from build123d import *

# Parameters (mm, degrees)
SKETCH5_W           = 26
SKETCH5_H           = 26
BOSS_EXTRUDE1_DEPTH = 10
SKETCH4_R           = 10.75
CUT_EXTRUDE1_DEPTH  = 4
SKETCH6_W           = 10
SKETCH6_H           = 3.483566845
CUT_EXTRUDE2_DEPTH  = 4
LPATTERN1_COUNT     = 8
LPATTERN1_PITCH     = 26
SKETCH7_W           = 10
SKETCH7_H           = 4
CUT_EXTRUDE3_DEPTH  = 183.737516674
SKETCH12_W          = 208
SKETCH12_H          = 10
BOSS_EXTRUDE3_DEPTH = 20
SKETCH14_W          = 46
SKETCH14_H          = 10
BOSS_EXTRUDE4_DEPTH = 20
SKETCH15_W          = 46
SKETCH15_H          = 20
BOSS_EXTRUDE5_DEPTH = 45
SKETCH16_W          = 20
SKETCH16_H          = 5
CUT_EXTRUDE5_DEPTH  = 20
SKETCH17_R          = 6
CUT_EXTRUDE6_DEPTH  = 45
SKETCH18_W          = 6
SKETCH18_H          = 19
CUT_EXTRUDE7_DEPTH  = 20
SNAP_START          = 2.145910006
SNAP_HOOK1_DEPTH    = 13
FILLET2_R           = 2


# Read off the part's stored shape, not the designer's step: Snap Hook1
with BuildPart() as part:
    # Sketch5 → Boss-Extrude1 (new body)
    with BuildSketch(Plane(origin=(0, 0, 0), x_dir=(1, 0, 0), z_dir=(0, 1, 0))):
        Rectangle(SKETCH5_W, SKETCH5_H)
    boss_extrude1 = extrude(amount=-BOSS_EXTRUDE1_DEPTH)

    # Sketch4 → Cut-Extrude1 (cut)
    with BuildSketch(Plane(origin=(0, 0, 0), x_dir=(1, 0, 0), z_dir=(0, 1, 0))):
        with Locations(Location((0, 0, 0), (0, 0, 270))):
            Circle(SKETCH4_R)
    cut_extrude1 = extrude(amount=-CUT_EXTRUDE1_DEPTH, mode=Mode.SUBTRACT)

    # Sketch6 → Cut-Extrude2 (cut)
    with BuildSketch(Plane(origin=(0, 0, 0), x_dir=(1, 0, 0), z_dir=(0, 1, 0))):
        with Locations((0, 11.258216578)):
            Rectangle(SKETCH6_W, SKETCH6_H)
    cut_extrude2 = extrude(amount=-CUT_EXTRUDE2_DEPTH, mode=Mode.SUBTRACT)

    # LPattern1: Boss-Extrude1, Cut-Extrude1, Cut-Extrude2 ×8
    with Locations(*[(0, 0, -i * LPATTERN1_PITCH) for i in range(1, LPATTERN1_COUNT)]):
        add(boss_extrude1)
        add(cut_extrude1, mode=Mode.SUBTRACT)
        add(cut_extrude2, mode=Mode.SUBTRACT)

    # Sketch7 → Cut-Extrude3 (cut, through all)
    with BuildSketch(Plane.XY.offset(-13)):
        with Locations((0, -2)):
            Rectangle(SKETCH7_W, SKETCH7_H)
    extrude(amount=-CUT_EXTRUDE3_DEPTH, mode=Mode.SUBTRACT)

    # Sketch12 → Boss-Extrude3 (add)
    with BuildSketch(Plane(origin=(13, 0, 0), x_dir=(0, 0, -1), z_dir=(1, 0, 0))):
        with Locations((91, -5)):
            Rectangle(SKETCH12_W, SKETCH12_H)
    extrude(amount=BOSS_EXTRUDE3_DEPTH)

    # Sketch14 → Boss-Extrude4 (add)
    with BuildSketch(Plane(origin=(0, 0, -195), x_dir=(-1, 0, 0), z_dir=(0, 0, -1))):
        with Locations((-10, -5)):
            Rectangle(SKETCH14_W, SKETCH14_H)
    extrude(amount=BOSS_EXTRUDE4_DEPTH)

    # Sketch15 → Boss-Extrude5 (add)
    with BuildSketch(Plane(origin=(0, 0, 0), x_dir=(1, 0, 0), z_dir=(0, 1, 0))):
        with Locations((10, 205)):
            Rectangle(SKETCH15_W, SKETCH15_H)
    extrude(amount=BOSS_EXTRUDE5_DEPTH)

    # Sketch16 → Cut-Extrude5 (cut)
    with BuildSketch(Plane(origin=(0, 0, -215), x_dir=(-1, 0, 0), z_dir=(0, 0, -1))):
        with Locations((0, -1.5)):
            Rectangle(SKETCH16_W, SKETCH16_H)
    extrude(amount=-CUT_EXTRUDE5_DEPTH, mode=Mode.SUBTRACT)

    # Sketch17 → Cut-Extrude6 (cut)
    with BuildSketch(Plane(origin=(0, 0, -215), x_dir=(-1, 0, 0), z_dir=(0, 0, -1))):
        with Locations((-0.602201255, 14)):
            Circle(SKETCH17_R)
    extrude(amount=-CUT_EXTRUDE6_DEPTH, mode=Mode.SUBTRACT)

    # Sketch18 → Cut-Extrude7 (cut)
    with BuildSketch(Plane.ZY.offset(13)):
        with Locations((-207, 13.5)):
            Rectangle(SKETCH18_W, SKETCH18_H)
    extrude(amount=-CUT_EXTRUDE7_DEPTH, mode=Mode.SUBTRACT)

    # Snap Hook1 outline → Snap Hook1 (add)
    with BuildSketch(Plane.YZ.offset(SNAP_START)):
        Polygon((45, -207.281762619), (65, -207.281762619), (65, -209.025762619), (71, -207.281762619), (71, -205.531762619), (45, -202.281762619), align=None)
    extrude(amount=SNAP_HOOK1_DEPTH)

    # Fillet2
    fillet2_edges = [part.edges().sort_by_distance(p)[0] for p in [
        (10, -10, -215),
        (10, -10, 13),
    ]]
    fillet(fillet2_edges, radius=FILLET2_R)


solid = part.part
The model under review builds one solid part; all positions refer to its coordinate system, in mm. A direction names the side the tool comes from. Round coordinates to 2 decimals unless told otherwise and drop trailing zeros. Loops run counter-clockwise (first coordinate to the right, second up) from the corner with the lowest first, then second, coordinate; pieces in that order, holes last. Notation, with made-up numbers: M -38,42 L -25,42 A4 cw -25,46 Z; hole C -39,86 d4. An arc over 180 degrees is marked long. Answer as CSV lines item,"result". Start each with the question number.
Item 1: For faces 1 (the face through (-10.75, -1.97, -26.16)), 2 (the face through (7, 14, -207)), 3 (the face through (0, 1, -205)), 4 (the face through (2.146, 55, -206)), list the 3-axis set-ups (+Z, -Z, +X, -X, +Y, -Y) from which the entire face can be reached by the end or side of a thin tool; tool diameter is ignored.
Item 2: Consider section B-B (x = 19.5). Write out the cut boundary in (y, z).
Item 3: Mouldability with a two-part tool opening along Y and no side actions: class faces 5 (the face through (15, 0, -90)), 6 (the face through (10.75, -1.97, -103.84)), 7 (the face through (10, -2, -205)) as released by +Y, released by -Y, zero draft, split by the parting line, or undercut.
Item 4: Wall thickness on line 1 (X direction, y = -0.95, z = 0); line 2 (Y direction, x = -2.5, z = -135.5); line 3 (Z direction, x = -5, y = 20): over which ranges is each line inside the solid? List them lowest first. Write a range as [from, to].
Item 5: Insertion check: P1, Ø3, axis at y = 14, z = -207, coming from the -X side; P2, Ø24.5, axis at x = 0, z = 0, coming from the +Y side; P3, Ø4, axis at x = -2, y = 43, coming from the +Z side. Each pin has a flat end and moves straight along its axis. Give the tip position at first contact, or say it passes through.
Item 6: Consider section D-D (x = 0). Write out the cut boundary in (y, z).
Item 7: Consider section A-A (y = 14). Write out the cut boundary in (x, z).
Item 8: Consider section C-C (z = 0). Write out the cut boundary in (x, y).
Answer:
1,face 1,"+Y"
1,face 2,"-X"
1,face 3,"+Z, -Z"
1,face 4,"+Z, -Z, -X, +Y"
2,outline,"M -10,-213 A2 ccw -8,-215 L 45,-215 L 45,-195 L 0,-195 L 0,13 L -8,13 A2 ccw -10,11 Z"
3,face 5,"released by +Y"
3,face 6,"zero draft"
3,face 7,"undercut"
4,line 1,"x = [-13, -10.75], [10.75, 33]"
4,line 2,"y = [-10, -4]"
4,line 3,"z = [-215, -210], [-204, -195]"
5,P1,"stops at x = 7"
5,P2,"stops at y = 0"
5,P3,"stops at z = -195"
6,outline,"M -10,-213 A2 ccw -8,-215 L -4,-215 L -4,10.75 L 0,10.75 L 0,13 L -8,13 A2 ccw -10,11 Z; M 1,-215 L 8.03,-215 L 8.03,-210 L 4,-210 L 4,-204 L 8.03,-204 L 8.03,-195 L 1,-195 Z; M 19.97,-215 L 45,-215 L 45,-195 L 19.97,-195 L 19.97,-204 L 23,-204 L 23,-210 L 19.97,-210 Z"
7,outline,"M -13,-215 L -5.4,-215 L -5.4,-210 L -13,-210 Z; M -13,-204 L -5.4,-204 L -5.4,-195 L -13,-195 Z; M 6.6,-215 L 33,-215 L 33,-195 L 6.6,-195 L 6.6,-204 L 7,-204 L 7,-210 L 6.6,-210 Z"
8,outline,"M -13,-10 L 33,-10 L 33,0 L 10.75,0 L 10.75,-4 L -10.75,-4 L -10.75,0 L -13,0 Z"
